Verification items for the finished model (mm, model axes). A direction names the side the tool comes from. Give positions to 0.01 mm unless a question says otherwise; leave off trailing zeros. Order: outer loops, then holes, each group sorted by start corner. A loop starts at its lowest first (then second) coordinate and runs counter-clockwise, first axis right, second up. Notation, with made-up numbers: (-29.75, -14) -> (22.25, -14) arc R36 ccw to (22.25, 21) -> close; hole circle Ø1 at (81.5, 23.25). An arc over 180 degrees is marked (long way). Write each question's results on one line, items separated by ' | '. Start each with the question number.
1. Material ranges on L1, parallel to X at y = 2.3, z = -61.5; L2, parallel to Z at x = -62, y = 1.3; L3, parallel to X at y = 2.6, z = -19.5, recorded low to high. Write a range as from..to.
2. Depth check by flat-ended pin: pin 1 Ø2 at (x, z) = (-0.5, -38.5) entering from +Y. Enter the tip coordinate at first touch or a pass-through.
3. Set-up check for faces 1 (the face through (-47, 3.175, -1)), 2 (the face through (-20.8, 1.6, 35.1)): record each of +Z, -Z, +X, -X, +Y, -Y from which the full face is reachable in a straight line by a thin tool's end or side.
4. Cross-section at A-A, the plane z = -7.5. Enter the section's corners in (x, y) (3 decimals), then the cut area to 3 significant figures.
5. Mould release check, pull along Z, two halves, no side actions. Record for faces 3 (the face through (-47, 0, -1)), 4 (the face through (-25.466, 1.565, 41.952)): +Z half, -Z half, draft (parallel to the pull), parting line (faces both ways), or undercut.
6. Cross-section at C-C, the plane x = 18. Enter the section's corners in (y, z) (3 decimals), then the cut area to 3 significant figures.
7. Cross-section at B-B, the plane y = 0.7. State how many separate pieces and enclosed holes the cut face has, then the cut area to 3 significant figures.
from build123d import *

# Parameters (mm, degrees)
SKETCH1_W             = 203
SKETCH1_H             = 138
BOSS_EXTRUDE1_DEPTH   = 3.175
F_3_0MM_DOWEL_HOLE1_D = 3
F_4_0MM_DOWEL_HOLE1_D = 4
CUT_EXTRUDE1_DEPTH    = 123.773493169


with BuildPart() as part:
    # Sketch1 → Boss-Extrude1 (new body)
    with BuildSketch(Plane(origin=(0, 0, 0), x_dir=(1, 0, 0), z_dir=(0, 1, 0))):
        Rectangle(SKETCH1_W, SKETCH1_H)
    extrude(amount=BOSS_EXTRUDE1_DEPTH)

    # Ø3.0mm Dowel Hole1 (through all)
    with Locations(Plane(origin=(0, 3.175, 0), x_dir=(1, 0, 0), z_dir=(0, 1, 0))):
        with Locations((-95.5, 61.5), (94.5, 61.5), (94.5, -61.5), (-95.5, -61.5), (-62, -46.6), (78, -45.5), (78, 47.5), (-62, 48.4)):
            Hole(F_3_0MM_DOWEL_HOLE1_D / 2)

    # Ø4.0mm Dowel Hole1 (through all)
    with Locations(Plane(origin=(0, 3.175, 0), x_dir=(1, 0, 0), z_dir=(0, 1, 0))):
        with Locations((-25.9, 40), (54.1, 40), (54.1, -40), (-25.9, -40)):
            Hole(F_4_0MM_DOWEL_HOLE1_D / 2)

    # Sketch7 → Cut-Extrude1 (cut, through all)
    with BuildSketch(Plane(origin=(0, 3.175, 0), x_dir=(1, 0, 0), z_dir=(0, 1, 0))):
        Polygon((-25.9, 30), (-15.9, 40), (44.1, 40), (54.1, 30), (54.1, -30), (44.1, -40), (-15.9, -40), (-25.9, -30), align=None)
    extrude(amount=-CUT_EXTRUDE1_DEPTH, mode=Mode.SUBTRACT)


solid = part.part
Results below:
1) L1: x = -101.5..-97, -94..93, 96..101.5 | L2: z = -69..-49.9, -46.9..45.1, 48.1..69 | L3: x = -101.5..-25.9, 54.1..101.5
2) pin 1: passes through
3) face 1: +Z, -Z, +X, -X, +Y | face 2: +Y, -Y
4) outline: (-101.5, 0) -> (-25.9, 0) -> (-25.9, 3.175) -> (-101.5, 3.175) -> close; (54.1, 0) -> (101.5, 0) -> (101.5, 3.175) -> (54.1, 3.175) -> close | area: 391 mm²
5) face 3: draft | face 4: undercut
6) outline: (0, -69) -> (3.175, -69) -> (3.175, -40) -> (0, -40) -> close; (0, 40) -> (3.175, 40) -> (3.175, 69) -> (0, 69) -> close | area: 184 mm²
7) separate pieces: 1 | enclosed holes: 13 | area: 21,700 mm²
